```python
from build123d import *

# Parameters (mm, degrees)
F0_W      = 27
F0_H      = 615
F1_DEPTH  = 20
F2_W      = 12
F2_H      = 20
F3_DEPTH  = 25
F4_W      = 12
F4_H      = 20
F5_DEPTH  = 33
F6_R      = 9.99999
F7_R      = 2.5
F8_DEPTH  = 30
F10_DEPTH = 25
F11_R     = 2.5
F12_DEPTH = 30
F14_DEPTH = 25
F15_R     = 1
F16_SIZE  = 3
F17_R     = 2


# Not quite as in the source:
# - a fillet or chamfer is up to 0.001 mm smaller than in the source, because OpenCascade refuses the exact size


with BuildPart() as f1:
    # F0 (on Front) → F1 (new body)
    with BuildSketch(Plane.XZ):
        Rectangle(F0_W, F0_H)
    extrude(amount=F1_DEPTH)

    # F2 (on face) → F3 (cut)
    with BuildSketch(Plane.XY.offset(307.5)):
        with Locations((0, -10)):
            Rectangle(F2_W, F2_H)
    extrude(amount=-F3_DEPTH, mode=Mode.SUBTRACT)

    # F4 (on face) → F5 (cut)
    with BuildSketch(Plane(origin=(0, 0, -307.5), x_dir=(1, 0, 0), z_dir=(0, 0, -1))):
        with Locations((0, 10)):
            Rectangle(F4_W, F4_H)
    extrude(amount=-F5_DEPTH, mode=Mode.SUBTRACT)

    # F6 (radius 10 in the source; OpenCascade refuses exactly that, so slightly less here)
    f6_edges = [f1.edges().sort_by_distance(p)[0] for p in [
        (-9.75, 0, -307.5),
        (9.75, 0, -307.5),
        (9.75, -20, -307.5),
        (-9.75, -20, -307.5),
        (-9.75, -20, 307.5),
        (-9.75, 0, 307.5),
        (9.75, 0, 307.5),
        (9.75, -20, 307.5),
    ]]
    fillet(f6_edges, radius=F6_R)

    # F7 (on face) → F8 (cut)
    with BuildSketch(Plane(origin=(-13.5, 0, 0), x_dir=(0, -1, 0), z_dir=(-1, 0, 0))):
        with Locations((10, 297.5)):
            Circle(F7_R)
        with Locations((10, -297.5)):
            Circle(F7_R)
    extrude(amount=-F8_DEPTH, mode=Mode.SUBTRACT)

    # F9 (on face) → F10 (cut)
    with BuildSketch(Plane.XZ.offset(20)):
        with BuildLine():
            ThreePointArc((9.5, -65), (0, -55.5), (-9.5, -65))
            Line((-9.5, -65), (-9.5, -180))
            ThreePointArc((-9.5, -180), (0, -189.5), (9.5, -180))
            Line((9.5, -180), (9.5, -65))
        make_face()
    extrude(amount=-F10_DEPTH, mode=Mode.SUBTRACT)

    # F11 (on face) → F12 (cut)
    with BuildSketch(Plane(origin=(-13.5, 0, 0), x_dir=(0, -1, 0), z_dir=(-1, 0, 0))):
        with Locations((10, -169.5)):
            Circle(F11_R)
    extrude(amount=-F12_DEPTH, mode=Mode.SUBTRACT)

    # F13 (on face) → F14 (cut)
    with BuildSketch(Plane.XZ.offset(20)):
        with BuildLine():
            ThreePointArc((7.5, 240), (0, 247.5), (-7.5, 240))
            Line((-7.5, 240), (-7.5, 40))
            ThreePointArc((-7.5, 40), (0, 32.5), (7.5, 40))
            Line((7.5, 40), (7.5, 240))
        make_face()
    extrude(amount=-F14_DEPTH, mode=Mode.SUBTRACT)

    # F15
    f15_edges = [f1.edges().sort_by_distance(p)[0] for p in [
        (13.5, -20, 0),
        (-13.5, -20, 0),
    ]]
    fillet(f15_edges, radius=F15_R)

    # F16
    f16_edges = [f1.edges().sort_by_distance(p)[0] for p in [
        (13.5, -7.5, 297.5),
        (13.5, -7.5, -169.5),
        (13.5, -7.5, -297.5),
    ]]
    chamfer(f16_edges, length=F16_SIZE)

    # F17
    f17_edges = [f1.edges().sort_by_distance(p)[0] for p in [
        (-6, -10, 282.5),
        (6, -10, 282.5),
        (6, -10, -274.5),
        (-6, -10, -274.5),
    ]]
    fillet(f17_edges, radius=F17_R)


solid = f1.part
```
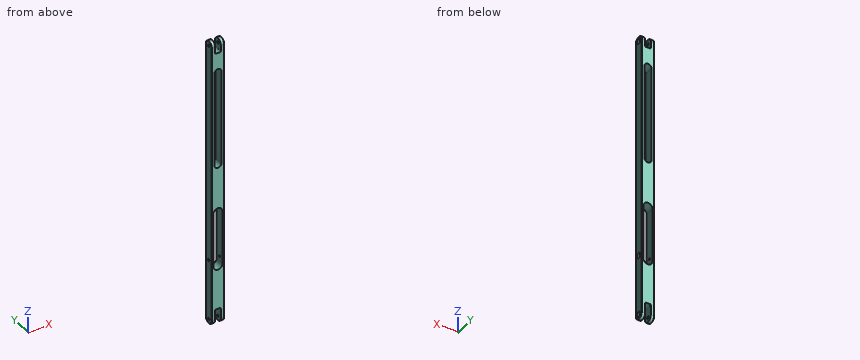
The listing builds one solid part. Answer for the finished solid, in the listing's coordinates (mm). Give positions to 0.01 mm unless a question says otherwise; leave off trailing zeros. Loops run counter-clockwise (first coordinate to the right, second up) from the corner with the lowest first, then second, coordinate; pieces in that order, holes last. Notation, with made-up numbers: (-5.75, 43) - (38.25, 43) arc R29 ccw to (38.25, 82) - close; hole circle Ø5 at (4.25, 33). An arc over 180 degrees is marked (long way). Return JSON: item names as keys, results as strings. Group by question number.
1. Straight lines are drawn through the part: line 1 (Y direction, x = 8.85, z = -297.5); line 2 (X direction, y = -11.5, z = 43.5); line 3 (X direction, y = -2.5, z = -150.5). For each, find the intervals that lie inside material, in ascending order. Write a range as [from, to].
2. Find section A-A (z = -133). Write down the section's boundary in (x, y).
3. Given pin 1 Ø6.5 at (y, z) = (-10, 297.5) entering from +X; pin 2 Ø9 at (x, y) = (-0.5, -11) entering from -Z; pin 3 Ø2 at (x, y) = (-5.5, -14) entering from -Z, each flat-ended and moving along its own axis, determine where each tip first touches the part or whether it passes through.
4. Find section B-B (z = 209). Write down the section's boundary in (x, y).
Verdict:
{
 "1": {"line 1": "y = [-20, -12.5], [-7.5, 0]", "line 2": "x = [-13.5, -7.5], [7.5, 13.5]", "line 3": "x = [-13.5, -9.5], [9.5, 13.5]"},
 "2": {"outline": "(-13.5, -19) arc R1 ccw to (-12.5, -20) - (-9.5, -20) - (-9.5, 0) - (-12.5, 0) arc R1 ccw to (-13.5, -1) - close; (9.5, -20) - (12.5, -20) arc R1 ccw to (13.5, -19) - (13.5, -1) arc R1 ccw to (12.5, 0) - (9.5, 0) - close"},
 "3": {"pin 1": "stops at x = 11.25", "pin 2": "stops at z = -274.77", "pin 3": "stops at z = -307"},
 "4": {"outline": "(-13.5, -19) arc R1 ccw to (-12.5, -20) - (-7.5, -20) - (-7.5, 0) - (-12.5, 0) arc R1 ccw to (-13.5, -1) - close; (7.5, -20) - (12.5, -20) arc R1 ccw to (13.5, -19) - (13.5, -1) arc R1 ccw to (12.5, 0) - (7.5, 0) - close"}
}
